from build123d import *

# Parameters (mm, degrees)
SKETCH3_W           = 38.1
SKETCH3_H           = 38.1
BOSS_EXTRUDE1_DEPTH = 2.286
SKETCH4_R           = 8.509
BOSS_EXTRUDE2_DEPTH = 22.86
DOME2_FACE_RADIUS   = 8.509
DOME2_HEIGHT        = 3.81


with BuildPart() as part:
    # Sketch3 → Boss-Extrude1 (new body)
    with BuildSketch(Plane(origin=(0, 0, 0), x_dir=(1, 0, 0), z_dir=(0, 1, 0))):
        Rectangle(SKETCH3_W, SKETCH3_H)
    extrude(amount=BOSS_EXTRUDE1_DEPTH)

    # Sketch4 → Boss-Extrude2 (add)
    with BuildSketch(Plane(origin=(0, 2.286, 0), x_dir=(1, 0, 0), z_dir=(0, 1, 0))):
        Circle(SKETCH4_R)
    extrude(amount=BOSS_EXTRUDE2_DEPTH)

    # Dome2: a dome of height H over a round flat face of radius A is a cap of a sphere of radius (A * A + H * H) / (2 * H)
    dome2_r = (DOME2_FACE_RADIUS * DOME2_FACE_RADIUS + DOME2_HEIGHT * DOME2_HEIGHT) / (2 * DOME2_HEIGHT)
    dome2_base = Plane((0, 25.146, 0), z_dir=(0, 1, 0))
    with Locations(dome2_base.offset(DOME2_HEIGHT - dome2_r)):
        dome2_ball = Sphere(dome2_r, mode=Mode.PRIVATE)
    add(split(dome2_ball, bisect_by=dome2_base, keep=Keep.TOP, mode=Mode.PRIVATE))


solid = part.part
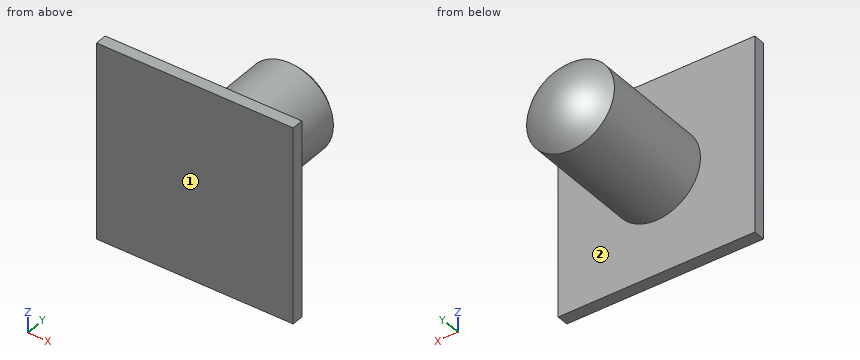
Geometry: final body of the model. Coordinates: model frame, mm. Face numbers are marked on the shaded views. A direction names the side the tool comes from. Round coordinates to 2 decimals unless told otherwise and drop trailing zeros. Order: outer loops, then holes, each group sorted by start corner. A loop starts at its lowest first (then second) coordinate and runs counter-clockwise, first axis right, second up.
Q1. Section A-A, the plane x = 0. Output: boundary loops of the cut face in (y, z).
Result sheet:
outline: (0, -19.05) - (2.29, -19.05) - (2.29, -8.51) - (25.15, -8.51) arc R11.41 ccw to (25.15, 8.51) - (2.29, 8.51) - (2.29, 19.05) - (0, 19.05) - close
Q2. Access query for the marked faces 1 and 2. Directions: +Z, -Z, +X, -X, +Y, -Y. A direction counts if a zero-diameter tool reaches every point of the face in a straight line with its end or side. Return the directions, or none.
Result sheet:
face 1: +Z, -Z, +X, -X, -Y
face 2: +Y
Q3. Pin query (flat end, axial travel): pin 1 (2 mm diameter, centred on x = 3.5, z = -5.5, fed in from +Y); pin 2 (6 mm diameter, centred on x = -12, z = -10, fed in from +Y); pin 3 (19 mm diameter, centred on x = -9.5, z = -1, fed in from +Y); pin 4 (4 mm diameter, centred on x = -12.5, y = 14.5, fed in from -Z). Return the tip coordinate at first contact, or that it passes through.
Result sheet:
pin 1: stops at y = 27.53
pin 2: stops at y = 2.29
pin 3: stops at y = 28.96
pin 4: passes through
Q4. Section D-D, the plane x = 11. Output: boundary loops of the cut face in (y, z).
Result sheet:
outline: (0, -19.05) - (2.29, -19.05) - (2.29, 19.05) - (0, 19.05) - close
Q5. Material intervals for probe 1 along Y at (x, z) = (16, 10); probe 2 along Z at (x, y) = (-7, 21.25); probe 3 along Y at (x, z) = (1.5, 6.5), sorted ascending.
Result sheet:
probe 1: y = 0 to 2.29
probe 2: z = -4.84 to 4.84
probe 3: y = 0 to 26.8
Q6. Section C-C, the plane y = 4. Output: boundary loops of the cut face in (x, z), and give its area (3 significant figures).
Result sheet:
outline: circle Ø17.02 at (0, 0)
area: 227 mm2
Q7. Section B-B, the plane z = 0. Output: boundary loops of the cut face in (x, y), and give its area (3 significant figures).
Result sheet:
outline: (-19.05, 0) - (19.05, 0) - (19.05, 2.29) - (8.51, 2.29) - (8.51, 25.15) arc R11.41 ccw to (-8.51, 25.15) - (-8.51, 2.29) - (-19.05, 2.29) - close
area: 521 mm2
